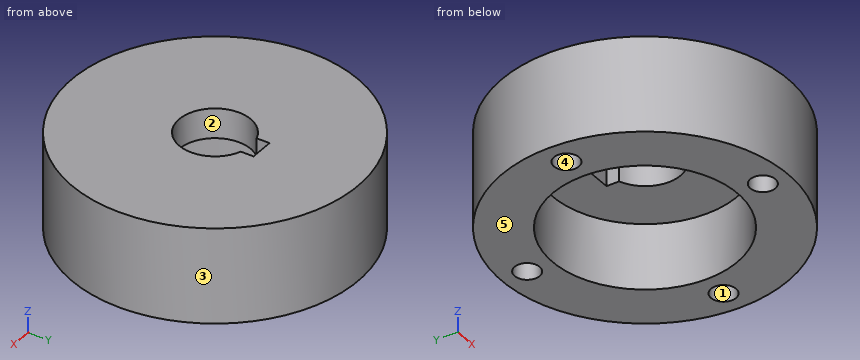
from build123d import *

# Parameters (mm, degrees)
SKETCH1_R                       = 24
BOSS_EXTRUDE1_DEPTH             = 5
BOSS_EXTRUDE2_START             = -11
SKETCH1_3_R                     = 24
SKETCH1_3_R_2                   = 15.5
BOSS_EXTRUDE2_DEPTH             = 11
TAP_DRILL_FOR_M5X0_8_TAP1_D     = 4.2
TAP_DRILL_FOR_M5X0_8_TAP1_DEPTH = 10
TAP_DRILL_FOR_M5X0_8_TAP1_TIP   = 1.2618073


with BuildPart() as part:
    # Sketch1 → Boss-Extrude1 (new body)
    with BuildSketch(Plane.XY):
        Circle(SKETCH1_R)
        with BuildLine():
            Line((-2, 5.656854249), (-2, 7.8))
            Line((-2, 7.8), (2, 7.8))
            Line((2, 7.8), (2, 5.656854249))
            ThreePointArc((2, 5.656854249), (0, -6), (-2, 5.656854249))
        make_face(mode=Mode.SUBTRACT)
    extrude(amount=BOSS_EXTRUDE1_DEPTH)

    # Sketch1<3> → Boss-Extrude2 (add)
    with BuildSketch(Plane.XY.offset(BOSS_EXTRUDE2_START)):
        Circle(SKETCH1_3_R)
        Circle(SKETCH1_3_R_2, mode=Mode.SUBTRACT)
    extrude(amount=BOSS_EXTRUDE2_DEPTH)

    # Tap Drill for M5x0.8 Tap1
    with Locations(Plane(origin=(0, 0, -11), x_dir=(-1, 0, 0), z_dir=(0, 0, -1))):
        with Locations((-19.75, 0), (0, -19.75), (19.75, 0), (0, 19.75)):
            Hole(TAP_DRILL_FOR_M5X0_8_TAP1_D / 2, depth=TAP_DRILL_FOR_M5X0_8_TAP1_DEPTH)
            with Locations((0, 0, -(TAP_DRILL_FOR_M5X0_8_TAP1_DEPTH + TAP_DRILL_FOR_M5X0_8_TAP1_TIP / 2))):  # 118° drill point
                Cone(0, TAP_DRILL_FOR_M5X0_8_TAP1_D / 2, TAP_DRILL_FOR_M5X0_8_TAP1_TIP, mode=Mode.SUBTRACT)


solid = part.part
CAD build for the part. Positions are in the model's coordinates, mm. Face numbers are marked on the shaded views. A direction names the side the tool comes from. Give positions to 0.01 mm unless a question says otherwise; leave off trailing zeros. Write each loop counter-clockwise with the first axis right and the second up, starting at its lowest first coordinate (ties: lowest second). Pieces come first, ordered by that corner, then holes. Notation, with made-up numbers: M -3.5,74.25 L 30.5,74.25 A31 cw 30.5,102.25 Z; hole C 30.5,31.25 d5. An arc over 180 degrees is marked long. Put each result on its own line as item: value. Start each with the question number.
(1) Mould opens along X. For the marked faces 3, 4 and 5 say: +X half, -X half, draft (parallel to the pull), parting line (faces both ways), or undercut.
(2) Flat gauge pins, fed straight in: pin 1 Ø8 at (x, z) = (-1.5, 1) entering from +Y; pin 2 Ø1 at (x, z) = (11.5, -6) entering from -Y; pin 3 Ø4 at (x, z) = (5, -8) entering from -Y. Where does each tip first touch, or does it go through?
(3) Band-saw the part on A-A, the plane y = 4. Write the cut outline in (x, z).
(4) Band-saw the part on B-B, the plane z = -7. Write the cut outline in (x, y).
(5) Which spindle directions (+Z, -Z, +X, -X, +Y, -Y) get a long thin tool onto all of the face, cutting with end or side? Do the marked faces 1 and 2. Say none if no direction does.
(6) Band-saw the part on D-D, the plane x = -11.5. Write the cut outline in (y, z).
(7) Probe L1, parallel to Y at x = 0, z = -4; L2, parallel to X at y = 1, z = -9.5; L3, parallel to Y at x = 0, z = 1.75. List the from-to ranges inside material, lowest first.
(8) Band-saw the part on C-C, the plane z = 1.5. Write the cut outline in (x, y), and give its area (3 significant figures).
Response values:
1. face 3: parting line
1. face 4: undercut
1. face 5: draft
2. pin 1: stops at y = 24
2. pin 2: stops at y = -21.33
2. pin 3: stops at y = -23.81
3. outline: M -23.66,-11 L -14.97,-11 L -14.97,0 L -4.47,0 L -4.47,5 L -23.66,5 Z; M 4.47,0 L 14.97,0 L 14.97,-11 L 23.66,-11 L 23.66,5 L 4.47,5 Z
4. outline: C 0,0 d48; hole C -19.75,0 d4.2; hole C 0,0 d31; hole C 0,-19.75 d4.2; hole C 0,19.75 d4.2; hole C 19.75,0 d4.2
5. face 1: -Z
5. face 2: +Z, -Z
6. outline: M -21.07,-11 L -10.39,-11 L -10.39,0 L 10.39,0 L 10.39,-11 L 21.07,-11 L 21.07,5 L -21.07,5 Z
7. L1: y = -24 to -21.85, -17.65 to -15.5, 15.5 to 17.65, 21.85 to 24
7. L2: x = -23.98 to -21.6, -17.9 to -15.47, 15.47 to 17.9, 21.6 to 23.98
7. L3: y = -24 to -6, 7.8 to 24
8. outline: C 0,0 d48; hole M -2,5.66 A6 ccw long 2,5.66 L 2,7.8 L -2,7.8 Z
8. area: 1,690 mm2
